The listing builds one solid part. Answer for the finished solid, in the listing's coordinates (mm). A direction names the side the tool comes from. Coordinates: 2 decimals unless noted, no trailing zeros. Write each loop counter-clockwise with the first axis right and the second up, starting at its lowest first coordinate (ties: lowest second). Pieces come first, ordered by that corner, then holes.
```python
from build123d import *

# Parameters (mm, degrees)
F2_W          = 7.7063473873
F2_H          = 14.5060643554
F3_DEPTH      = 29.9826746265
F3_DEPTH_BACK = 25.4
F4_W          = 6.6132526845
F4_H          = 12.692797929
F5_DEPTH      = 29.9826746265
F5_DEPTH_BACK = 25.4


with BuildPart() as f1:
    # F0 (on Front) → F1 (revolve)
    with BuildSketch(Plane.XZ):
        Polygon((0, -61.5766718984), (0, 24.0749828517), (-15.0857353583, 24.0749828517), (-15.0857353583, 31.7712202668), (-21.5406417847, 31.7712202668), (-21.5406417847, 12.4064972624), (-18.5614544898, 8.9307781309), (-10.120421648, 6.6963867284), (-8.1342970952, 4.2137298733), (-10.120421648, 2.6248309761), (-10.120421648, 0), (-8.1342970952, -3.7307715975), (-10.120421648, -41.9636853039), (-15.0857353583, -45.4394035041), (-21.0441108793, -45.4394035041), (-26.7542209476, -49.163389951), (-29.9816746265, -55.6182973087), (-29.9816746265, -61.5766718984), align=None)
    revolve(axis=Axis((0, 0, -18.7508445233), (0, 0, 1)))

    # F2 (on Front) → F3 (cut, two sides)
    with BuildSketch(Plane.XZ) as f3_sk:
        with Locations((0, 32.1853272617)):
            Rectangle(F2_W, F2_H)
    extrude(amount=-F3_DEPTH, mode=Mode.SUBTRACT)
    extrude(f3_sk.sketch, amount=F3_DEPTH_BACK, mode=Mode.SUBTRACT)

    # F4 (on Right) → F5 (cut, two sides)
    with BuildSketch(Plane.YZ) as f5_sk:
        with Locations((0, 31.875140965)):
            Rectangle(F4_W, F4_H)
    extrude(amount=F5_DEPTH, mode=Mode.SUBTRACT)
    extrude(f5_sk.sketch, amount=-F5_DEPTH_BACK, mode=Mode.SUBTRACT)


solid = f1.part
```
(1) Which of the six approach directions +Z, -Z, +X, -X, +Y, -Y give full straight-line access (tool end or side, diameter ignored) to faces 1 (the flat face through (0, -18, 24.932)), 2 (the flat face through (18, -3.307, 29)), 3 (the conical face through (-7.85, -2.47, -3.55))?
(2) Each of these flat-tipped pins is pushed along its axis until it touches: pin 1 (10 mm diameter, centred on x = -20, z = 19, fed in from -Y); pin 2 (5.5 mm diameter, centred on y = 16.5, z = 26.5, fed in from -X); pin 3 (12 mm diameter, centred on x = 16, z = -23, fed in from +Y); pin 4 (2 mm diameter, centred on y = -16.5, z = 27.5, fed in from -X). Where does it stop, or does it pass through?
(3) Section D-D, the plane z = -6 is taken. Write down the section's boundary in (x, y), plus the area to 3 significant figures.
(4) Find the intervals of material crossed by probe 1 along Z at (x, y) = (11, -3.5); probe 2 along Z at (x, y) = (-12, -17); probe 3 along Z at (x, y) = (20, 12), in increasing order.
(5) Section C-C, the plane z = 15 is taken. Write down the section's boundary in (x, y).
(6) For a pull along Z with two mould halves and no side action, classify faces 4 (the cylindrical face through (-9.653, -3.04, 1.294)), 5 (the flat face through (-13, -12, 31.771)), 6 (the flat face through (-18, -3.307, 29)) as pulls with the +Z half, pulls with the -Z half, needs draft (parallel to the pull), parting line crosses it, or undercut.
Solution:
1. face 1: +Z, +Y, -Y
1. face 2: +Z, +X, -X
1. face 3: none
2. pin 1: stops at y = -15.46
2. pin 2: stops at x = -16.58
2. pin 3: passes through
2. pin 4: stops at x = -14.96
3. outline: circle Ø16.5 at (0, 0)
3. area: 214 mm2
4. probe 1: z = -61.58 to -42.96, 7.07 to 24.07
4. probe 2: z = -61.58 to -45.44, 11.55 to 31.77
4. probe 3: z = -61.58 to -46.93
5. outline: circle Ø43.08 at (0, 0)
6. face 4: undercut
6. face 5: pulls with the +Z half
6. face 6: needs draft
